Work out the finished part from the listing and answer in its coordinate system (mm). Face numbers are marked on the shaded views. A direction names the side the tool comes from. Give positions to 0.01 mm unless a question says otherwise; leave off trailing zeros. Loops run counter-clockwise (first coordinate to the right, second up) from the corner with the lowest first, then second, coordinate; pieces in that order, holes last. Notation, with made-up numbers: M 77.25,-12.5 L 132.25,-12.5 A16 ccw 132.25,5.5 Z; hole C -24.75,6.5 d9. An arc over 180 degrees is marked long. Use a Markdown table: item, result.
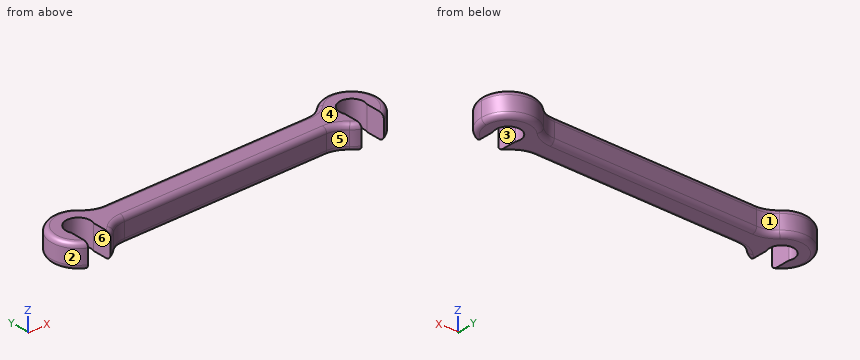
```python
from build123d import *

# Parameters (mm, degrees)
F0_R     = 2.5
F1_DEPTH = 5
F2_R     = 5
F3_R     = 1
F4_W     = 4.6
F4_H     = 8.970495
F5_DEPTH = 5.001


with BuildPart() as f1:
    # F0 (on Top) → F1 (new body)
    with BuildSketch(Plane.XY):
        with BuildLine():
            ThreePointArc((23.351021, -2.5), (29.535615, -5.347634), (33.75, 0))
            ThreePointArc((33.75, 0), (29.535615, 5.347634), (23.351021, 2.5))
            ThreePointArc((23.351021, 2.5), (22.75, 0), (23.351021, -2.5))
        make_face()
        with Locations((28.25, 0)):
            Circle(F0_R, mode=Mode.SUBTRACT)
        with BuildLine():
            ThreePointArc((23.351021, -2.5), (22.75, 0), (23.351021, 2.5))
            Line((23.351021, 2.5), (-23.351021, 2.5))
            ThreePointArc((-23.351021, 2.5), (-22.902366, 1.285615), (-22.75, 0))
            ThreePointArc((-22.75, 0), (-22.902366, -1.285615), (-23.351021, -2.5))
            Line((-23.351021, -2.5), (23.351021, -2.5))
        make_face()
        with BuildLine():
            ThreePointArc((-22.75, 0), (-22.902366, 1.285615), (-23.351021, 2.5))
            ThreePointArc((-23.351021, 2.5), (-33.75, 0), (-23.351021, -2.5))
            ThreePointArc((-23.351021, -2.5), (-22.902366, -1.285615), (-22.75, 0))
        make_face()
        with Locations((-28.25, 0)):
            Circle(F0_R, mode=Mode.SUBTRACT)
    extrude(amount=F1_DEPTH)

    # F2
    f2_edges = [f1.edges().sort_by_distance(p)[0] for p in [
        (-23.351021, -2.5, 2.5),
        (-23.351021, 2.5, 2.5),
        (23.351021, 2.5, 2.5),
        (23.351021, -2.5, 2.5),
    ]]
    fillet(f2_edges, radius=F2_R)

    # F3
    f3_edges = [f1.edges().sort_by_distance(p)[0] for p in [
        (0, -2.5, 5),
        (0, -2.5, 0),
    ]]
    fillet(f3_edges, radius=F3_R)

    # F4 (on Top) → F5 (cut, through all)
    with BuildSketch(Plane.XY):
        with Locations((-28.25, -4.485247)):
            Rectangle(F4_W, F4_H)
        with Locations((28.25, -4.485247)):
            Rectangle(F4_W, F4_H)
    extrude(amount=F5_DEPTH, mode=Mode.SUBTRACT)


solid = f1.part
```
(1) The mould has two halves that part along X. Classify the marked faces 4, 5 and 6: released by +X, released by -X, zero draft, split by the parting line, or undercut.
Entries:
| item | result |
|---|---|
| face 4 | zero draft |
| face 5 | undercut |
| face 6 | undercut |
(2) A cutting plane is placed at B-B (z = 3.4). Write down the section's boundary in (x, y).
Entries:
| item | result |
|---|---|
| outline | M -30.55,-5 L -30.55,-0.98 A2.5 cw long -25.95,-0.98 L -25.95,-5 A5.5 ccw -24.4,-3.93 A5 cw -20.9,-2.5 L 20.9,-2.5 A5 cw 24.4,-3.93 A5.5 ccw 25.95,-5 L 25.95,-0.98 A2.5 cw long 30.55,-0.98 L 30.55,-5 A5.5 ccw long 24.4,3.93 A5 cw 20.9,2.5 L -20.9,2.5 A5 cw -24.4,3.93 A5.5 ccw long Z |
(3) Consider probe 1 along X at (y, z) = (1.5, 1.9); probe 2 along X at (y, z) = (0.5, 0.9); probe 3 along Y at (x, z) = (-15.5, 2.45). Determine where each line is inside the solid, lowest interval first. Write a range as [from, to].
Entries:
| item | result |
|---|---|
| probe 1 | x = [-33.54, -30.25], [-26.25, 26.25], [30.25, 33.54] |
| probe 2 | x = [-33.72, -30.7], [-25.8, 25.8], [30.7, 33.72] |
| probe 3 | y = [-2.5, 2.5] |
(4) Given P1, Ø1.2, axis at y = -3.5, z = 3, coming from the -X side; P2, Ø4.5, axis at x = 28.25, y = 0, coming from the +Z side; P3, Ø1, axis at y = 2.5, z = 3, coming from the +X side; P4, Ø3, axis at x = 9.5, z = 0.5, coming from the -Y side, each flat-ended and moving along its own axis, determine where each tip first touches the part or whether it passes through.
Entries:
| item | result |
|---|---|
| P1 | stops at x = -32.92 |
| P2 | passes through |
| P3 | stops at x = 33.37 |
| P4 | stops at y = -2.5 |
(5) Which of the six approach directions +Z, -Z, +X, -X, +Y, -Y give full straight-line access (tool end or side, diameter ignored) to the marked faces 1, 2 and 3?
Entries:
| item | result |
|---|---|
| face 1 | +Z, -Z, +Y |
| face 2 | +Z, -Z |
| face 3 | +Z, -Z, -Y |
(6) A cutting plane is placed at A-A (x = 8). Write down the section's boundary in (y, z), and give its area (3 significant figures).
Entries:
| item | result |
|---|---|
| outline | M -2.5,1 A1 ccw -1.5,0 L 1.5,0 A1 ccw 2.5,1 L 2.5,4 A1 ccw 1.5,5 L -1.5,5 A1 ccw -2.5,4 Z |
| area | 24.1 mm² |
